The model under review builds one solid part; all positions refer to its coordinate system, in mm. Round coordinates to 2 decimals unless told otherwise and drop trailing zeros. Loops run counter-clockwise (first coordinate to the right, second up) from the corner with the lowest first, then second, coordinate; pieces in that order, holes last. Notation, with made-up numbers: M -4.5,-22.75 L 45.5,-22.75 A37 cw 45.5,16.25 Z; hole C -10,76.5 d4. An arc over 180 degrees is marked long. Answer in a Markdown table with one row per item. Add a question column.
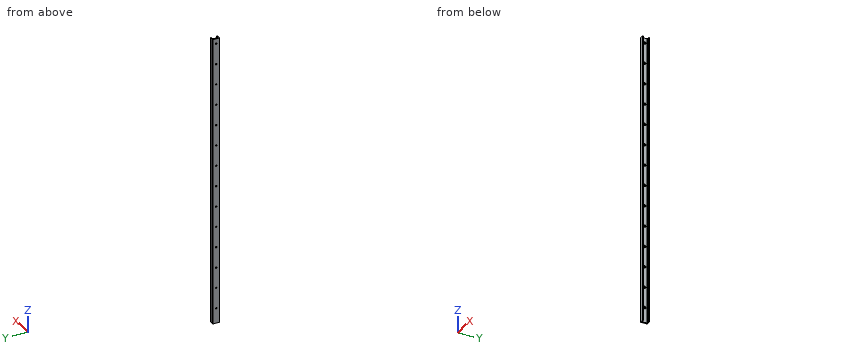
from build123d import *

# Parameters (mm, degrees)
BOSS_EXTRUDE1_DEPTH = 1219.2
SKETCH2_R           = 4.8895
CUT_EXTRUDE1_DEPTH  = 2.794
SKETCH3_R           = 2.8956
CUT_EXTRUDE2_DEPTH  = 1220.345961888
LPATTERN1_COUNT     = 31
LPATTERN1_PITCH     = 80
CUT_EXTRUDE3_START  = -1320.8
CUT_EXTRUDE3_DEPTH  = 1320.8


with BuildPart() as part:
    # Sketch1 → Boss-Extrude1 (new, symmetric)
    with BuildSketch(Plane.XY):
        with BuildLine():
            Line((15.494, 12.954), (4.394, 12.954))
            ThreePointArc((4.394, 12.954), (4.064, 12.624), (3.734, 12.954))
            Line((3.734, 12.954), (1.016, 12.954))
            ThreePointArc((1.016, 12.954), (0.29757951, 12.65642049), (0, 11.938))
            Line((0, 11.938), (0, -11.938))
            ThreePointArc((0, -11.938), (0.29757951, -12.65642049), (1.016, -12.954))
            Line((1.016, -12.954), (13.97, -12.954))
            ThreePointArc((13.97, -12.954), (14.68842049, -12.65642049), (14.986, -11.938))
            Line((14.986, -11.938), (14.986, -10.832020833))
            ThreePointArc((14.986, -10.832020833), (14.920380976, -10.472810588), (14.732, -10.16))
            Line((14.732, -10.16), (6.604, -10.16))
            ThreePointArc((6.604, -10.16), (5.86023638, -9.41623638), (5.588, -8.40023638))
            Line((5.588, -8.40023638), (5.588, 8.40023638))
            ThreePointArc((5.588, 8.40023638), (5.86023638, 9.41623638), (6.604, 10.16))
            Line((6.604, 10.16), (14.732, 10.16))
            ThreePointArc((14.732, 10.16), (15.853210245, 9.881639857), (16.51, 10.832020833))
            Line((16.51, 10.832020833), (16.51, 11.938))
            ThreePointArc((16.51, 11.938), (16.21242049, 12.65642049), (15.494, 12.954))
        make_face()
    extrude(amount=BOSS_EXTRUDE1_DEPTH, both=True)

    # Sketch2 → Cut-Extrude1 (cut)
    with BuildSketch(Plane(origin=(5.588, 0, 0), x_dir=(0, 0, -1), z_dir=(1, 0, 0))):
        with Locations(Location((-1200, 0, 0), (0, 0, 90))):
            Circle(SKETCH2_R)
    cut_extrude1 = extrude(amount=-CUT_EXTRUDE1_DEPTH, mode=Mode.SUBTRACT)

    # Sketch3 → Cut-Extrude2 (cut, through all)
    with BuildSketch(Plane(origin=(2.794, 0, 0), x_dir=(0, 0, -1), z_dir=(1, 0, 0))):
        with Locations(Location((-1200, 0, 0), (0, 0, 90))):
            Circle(SKETCH3_R)
    cut_extrude2 = extrude(amount=-CUT_EXTRUDE2_DEPTH, mode=Mode.SUBTRACT)

    # LPattern1: Cut-Extrude1, Cut-Extrude2 ×31
    with Locations(*[(0, 0, -i * LPATTERN1_PITCH) for i in range(1, LPATTERN1_COUNT)]):
        add(cut_extrude1, mode=Mode.SUBTRACT)
        add(cut_extrude2, mode=Mode.SUBTRACT)

    # Sketch5 → Cut-Extrude3 (cut)
    with BuildSketch(Plane(origin=(0, 0, -1219.2), x_dir=(-1, 0, 0), z_dir=(0, 0, -1)).offset(CUT_EXTRUDE3_START)):
        with BuildLine():
            Line((-16.51, 11.938), (-16.51, 10.832020833))
            ThreePointArc((-16.51, 10.832020833), (-15.853210245, 9.881639857), (-14.732, 10.16))
            Line((-14.732, 10.16), (-6.604, 10.16))
            ThreePointArc((-6.604, 10.16), (-5.86023638, 9.41623638), (-5.588, 8.40023638))
            Line((-5.588, 8.40023638), (-5.588, -8.40023638))
            ThreePointArc((-5.588, -8.40023638), (-5.86023638, -9.41623638), (-6.604, -10.16))
            Line((-6.604, -10.16), (-14.732, -10.16))
            ThreePointArc((-14.732, -10.16), (-14.920380976, -10.472810588), (-14.986, -10.832020833))
            Line((-14.986, -10.832020833), (-14.986, -11.938))
            ThreePointArc((-14.986, -11.938), (-14.68842049, -12.65642049), (-13.97, -12.954))
            Line((-13.97, -12.954), (-1.016, -12.954))
            ThreePointArc((-1.016, -12.954), (-0.29757951, -12.65642049), (0, -11.938))
            Line((0, -11.938), (0, 11.938))
            ThreePointArc((0, 11.938), (-0.29757951, 12.65642049), (-1.016, 12.954))
            Line((-1.016, 12.954), (-3.734, 12.954))
            ThreePointArc((-3.734, 12.954), (-4.064, 12.624), (-4.394, 12.954))
            Line((-4.394, 12.954), (-15.494, 12.954))
            ThreePointArc((-15.494, 12.954), (-16.21242049, 12.65642049), (-16.51, 11.938))
        make_face()
    extrude(amount=CUT_EXTRUDE3_DEPTH, mode=Mode.SUBTRACT)


solid = part.part
1. Take a section at B-B, the plane z = 656. State the section outline as (x, y) points, and give its area (3 significant figures).
2. To check wall thickness, follow probe 1 along Y at (x, z) = (4.35, 400); probe 2 along Y at (x, z) = (12.75, 149.5); probe 3 along X at (y, z) = (7, 492). State the ranges of each line that lie inside material, in increasing order.
3. For pin 1 Ø4.5 at (y, z) = (0, 400) entering from +X; pin 2 Ø11 at (y, z) = (1.5, 638.5) entering from +X; pin 3 Ø5 at (y, z) = (0.5, 1201) entering from +X; pin 4 Ø1.2 at (y, z) = (-11.5, 677) entering from +X, all flat-tipped, find the tip position at first contact; note any pin that passes through.
4. Take a section at A-A, the plane x = 9.5. State the section outline as (y, z) points.
Check sheet entries:
| question | item | result |
|---|---|---|
| 1 | outline | M 0,-11.94 A1.02 ccw 1.02,-12.95 L 13.97,-12.95 A1.02 ccw 14.99,-11.94 L 14.99,-10.83 A1.02 ccw 14.73,-10.16 L 6.6,-10.16 A2.03 cw 5.59,-8.4 L 5.59,8.4 A2.03 cw 6.6,10.16 L 14.73,10.16 A1.02 ccw 16.51,10.83 L 16.51,11.94 A1.02 ccw 15.49,12.95 L 4.39,12.95 A0.33 cw 3.73,12.95 L 1.02,12.95 A1.02 ccw 0,11.94 Z |
| 1 | area | 202 mm^2 |
| 2 | probe 1 | y = -12.95 to -4.89, 4.89 to 12.79 |
| 2 | probe 2 | y = -12.95 to -10.16, 10.16 to 12.95 |
| 2 | probe 3 | x = 0 to 5.59 |
| 3 | pin 1 | passes through |
| 3 | pin 2 | stops at x = 5.59 |
| 3 | pin 3 | stops at x = 2.79 |
| 3 | pin 4 | stops at x = 14.99 |
| 4 | outline | M -12.95,101.6 L -10.16,101.6 L -10.16,1219.2 L -12.95,1219.2 Z; M 10.16,101.6 L 12.95,101.6 L 12.95,1219.2 L 10.16,1219.2 Z |
